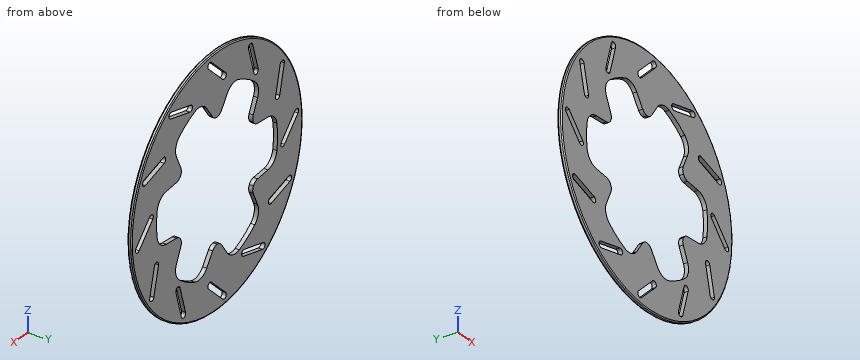
```python
from build123d import *

# Parameters (mm, degrees)
F0_R     = 120
F1_DEPTH = 4
F2_R     = 1
F3_R     = 1


# Not quite as in the source:
# - ends of sketch curves that miss each other by under 0.0002 mm in the source are joined


with BuildPart() as f1:
    # F0 (on Front) → F1 (new body)
    with BuildSketch(Plane.XZ):
        with Locations((0.769432, 5.271099)):
            Circle(F0_R)
        with BuildLine():
            ThreePointArc((-62.9582121085, -89.2513825538), (-66.5821895538, -87.0453028915), (-64.3761098915, -83.4213254462))
            Line((-64.3761098915, -83.4213254462), (-37.509664, -76.887277))
            ThreePointArc((-37.509664, -76.887277), (-33.8856864462, -79.0933561085), (-36.0917661085, -82.7173335538))
            Line((-36.0917661085, -82.7173335538), (-62.9582121085, -89.2513825538))
        make_face(mode=Mode.SUBTRACT)
        with BuildLine():
            ThreePointArc((-101.6815671027, -44.7239493504), (-103.7169843504, -41.0014398973), (-99.9944748973, -38.9660226496))
            Line((-99.9944748973, -38.9660226496), (-73.460425, -46.740593))
            ThreePointArc((-73.460425, -46.740593), (-71.4250076496, -50.4631031027), (-75.1475171027, -52.4985203504))
            Line((-75.1475171027, -52.4985203504), (-101.6815671027, -44.7239493504))
        make_face(mode=Mode.SUBTRACT)
        with BuildLine():
            ThreePointArc((-112.9532601885, 13.1996168201), (-112.8547281799, 17.4411131885), (-108.6132318115, 17.3425811799))
            Line((-108.6132318115, 17.3425811799), (-89.521356, -2.657419))
            ThreePointArc((-89.521356, -2.657419), (-89.6198878201, -6.8989151885), (-93.8613841885, -6.8003831799))
            Line((-93.8613841885, -6.8003831799), (-112.9532601885, 13.1996168201))
        make_face(mode=Mode.SUBTRACT)
        with BuildLine():
            ThreePointArc((-7.1590858201, -108.4515931885), (-11.4005821885, -108.3530611799), (-11.3020501799, -104.1115648115))
            Line((-11.3020501799, -104.1115648115), (8.69795, -85.019689))
            ThreePointArc((8.69795, -85.019689), (12.9394461885, -85.1182218201), (12.8409141799, -89.3597181885))
            Line((12.8409141799, -89.3597181885), (-7.1590858201, -108.4515931885))
        make_face(mode=Mode.SUBTRACT)
        with BuildLine():
            ThreePointArc((50.7644803504, -97.1799001027), (47.0419708973, -99.2153173504), (45.0065536496, -95.4928078973))
            Line((45.0065536496, -95.4928078973), (52.781124, -68.958759))
            ThreePointArc((52.781124, -68.958759), (56.5036341027, -66.9233416496), (58.5390513504, -70.6458511027))
            Line((58.5390513504, -70.6458511027), (50.7644803504, -97.1799001027))
        make_face(mode=Mode.SUBTRACT)
        with BuildLine():
            ThreePointArc((95.2919145538, -58.4565451085), (93.0858348915, -62.0805225538), (89.4618574462, -59.8744428915))
            Line((89.4618574462, -59.8744428915), (82.927808, -33.007997))
            ThreePointArc((82.927808, -33.007997), (85.1338871085, -29.3840194462), (88.7578645538, -31.5900991085))
            Line((88.7578645538, -31.5900991085), (95.2919145538, -58.4565451085))
        make_face(mode=Mode.SUBTRACT)
        with BuildLine():
            ThreePointArc((114.4921251885, -2.6574188201), (114.3935931799, -6.8989151885), (110.1520968115, -6.8003831799))
            Line((110.1520968115, -6.8003831799), (91.060221, 13.199617))
            ThreePointArc((91.060221, 13.199617), (91.1587528201, 17.4411131885), (95.4002491885, 17.3425811799))
            Line((95.4002491885, 17.3425811799), (114.4921251885, -2.6574188201))
        make_face(mode=Mode.SUBTRACT)
        with BuildLine():
            ThreePointArc((-93.7530495538, 68.9987431085), (-91.5469698915, 72.6227205538), (-87.9229924462, 70.4166408915))
            Line((-87.9229924462, 70.4166408915), (-81.388943, 43.550195))
            ThreePointArc((-81.388943, 43.550195), (-83.5950221085, 39.9262174462), (-87.2189995538, 42.1322971085))
            Line((-87.2189995538, 42.1322971085), (-93.7530495538, 68.9987431085))
        make_face(mode=Mode.SUBTRACT)
        with BuildLine():
            ThreePointArc((-49.2256163504, 107.7220981027), (-45.5031068973, 109.7575153504), (-43.4676896496, 106.0350058973))
            Line((-43.4676896496, 106.0350058973), (-51.24226, 79.500956))
            ThreePointArc((-51.24226, 79.500956), (-54.9647691027, 77.4655396496), (-57.0001863504, 81.1880491027))
            Line((-57.0001863504, 81.1880491027), (-49.2256163504, 107.7220981027))
        make_face(mode=Mode.SUBTRACT)
        with BuildLine():
            ThreePointArc((15.296097835, 79.396963116), (22.7229925826, 84.7551105395), (31.8731110928, 84.3758472359))
            ThreePointArc((31.8731110928, 84.3758472359), (43.2694321028, 78.8832582623), (53.724314001, 71.7600490012))
            ThreePointArc((53.724314001, 71.7600490012), (58.6278254217, 64.0254452963), (57.7009806311, 54.9144921712))
            Line((57.7009806311, 54.9144921712), (51.557275, 41.678832))
            ThreePointArc((51.557275, 41.678832), (50.8675495212, 38.1873960638), (51.8649313537, 34.7710992042))
            ThreePointArc((51.8649313537, 34.7710992042), (54.3248400002, 32.1991927067), (57.6933760416, 31.0507944662))
            Line((57.6933760416, 31.0507944662), (72.227646, 29.753569))
            ThreePointArc((72.227646, 29.753569), (80.5813855597, 26.0007639127), (84.8279934344, 17.8868970652))
            ThreePointArc((84.8279934344, 17.8868970652), (85.769432, 5.271099), (84.8279927873, -7.3446989681))
            ThreePointArc((84.8279927873, -7.3446989681), (80.5813855597, -15.4585659127), (72.2276460446, -19.2113714997))
            Line((72.2276460446, -19.2113714997), (57.693376, -20.508597))
            ThreePointArc((57.693376, -20.508597), (54.3248400002, -21.6569947067), (51.8649313537, -24.2289012042))
            ThreePointArc((51.8649313537, -24.2289012042), (50.8675495212, -27.6451980638), (51.5572758618, -31.1366350642))
            Line((51.5572758618, -31.1366350642), (57.700981, -44.372294))
            ThreePointArc((57.700981, -44.372294), (58.6278254217, -53.4832472963), (53.7243149172, -61.217850896))
            ThreePointArc((53.7243149172, -61.217850896), (43.2694321028, -68.3410602623), (31.8731109925, -73.833648981))
            ThreePointArc((31.8731109925, -73.833648981), (22.7229925826, -74.2129125395), (15.296097835, -68.854765116))
            Line((15.296097835, -68.854765116), (6.905533, -56.91633))
            ThreePointArc((6.905533, -56.91633), (4.2267227516, -54.5732912865), (0.769432, -53.728901))
            ThreePointArc((0.769432, -53.728901), (-2.6878587516, -54.5732912865), (-5.3666687757, -56.9163301576))
            Line((-5.3666687757, -56.9163301576), (-13.757233, -68.854765))
            ThreePointArc((-13.757233, -68.854765), (-21.1841275826, -74.2129125395), (-30.3342460928, -73.8336492359))
            ThreePointArc((-30.3342460928, -73.8336492359), (-41.7305681028, -68.3410602623), (-52.185450001, -61.2178510012))
            ThreePointArc((-52.185450001, -61.2178510012), (-57.0889604217, -53.4832472963), (-56.1621156311, -44.3722941712))
            Line((-56.1621156311, -44.3722941712), (-50.018411, -31.136635))
            ThreePointArc((-50.018411, -31.136635), (-49.3286845212, -27.6451980638), (-50.3260663537, -24.2289012042))
            ThreePointArc((-50.3260663537, -24.2289012042), (-52.7859750002, -21.6569947067), (-56.1545110416, -20.5085964662))
            Line((-56.1545110416, -20.5085964662), (-70.688781, -19.211372))
            ThreePointArc((-70.688781, -19.211372), (-79.0425205597, -15.4585659127), (-83.2891284344, -7.3446990652))
            ThreePointArc((-83.2891284344, -7.3446990652), (-84.230568, 5.271099), (-83.2891287873, 17.8868969681))
            ThreePointArc((-83.2891287873, 17.8868969681), (-79.0425205597, 26.0007639127), (-70.6887810446, 29.7535694997))
            Line((-70.6887810446, 29.7535694997), (-56.154511, 31.050794))
            ThreePointArc((-56.154511, 31.050794), (-52.7859750002, 32.1991927067), (-50.3260663537, 34.7710992042))
            ThreePointArc((-50.3260663537, 34.7710992042), (-49.3286845212, 38.1873960638), (-50.0184108618, 41.6788330642))
            Line((-50.0184108618, 41.6788330642), (-56.162116, 54.914492))
            ThreePointArc((-56.162116, 54.914492), (-57.0889604217, 64.0254452963), (-52.1854499172, 71.760048896))
            ThreePointArc((-52.1854499172, 71.760048896), (-41.7305681028, 78.8832582623), (-30.3342469925, 84.375846981))
            ThreePointArc((-30.3342469925, 84.375846981), (-21.1841275826, 84.7551105395), (-13.757232835, 79.396963116))
            Line((-13.757232835, 79.396963116), (-5.366668, 67.458528))
            ThreePointArc((-5.366668, 67.458528), (-2.6878587516, 65.1154892865), (0.769432, 64.271099))
            ThreePointArc((0.769432, 64.271099), (4.2267227516, 65.1154892865), (6.9055327757, 67.4585281576))
            Line((6.9055327757, 67.4585281576), (15.296097835, 79.396963116))
        make_face(mode=Mode.SUBTRACT)
        with BuildLine():
            ThreePointArc((103.2204321027, 55.2661473504), (105.2558493504, 51.5436378973), (101.5333398973, 49.5082206496))
            Line((101.5333398973, 49.5082206496), (74.99929, 57.282791))
            ThreePointArc((74.99929, 57.282791), (72.9638726496, 61.0053001027), (76.6863821027, 63.0407173504))
            Line((76.6863821027, 63.0407173504), (103.2204321027, 55.2661473504))
        make_face(mode=Mode.SUBTRACT)
        with BuildLine():
            ThreePointArc((64.4970771085, 99.7935805538), (68.1210545538, 97.5875008915), (65.9149748915, 93.9635234462))
            Line((65.9149748915, 93.9635234462), (39.048529, 87.429474))
            ThreePointArc((39.048529, 87.429474), (35.4245514462, 89.6355541085), (37.6306311085, 93.2595315538))
            Line((37.6306311085, 93.2595315538), (64.4970771085, 99.7935805538))
        make_face(mode=Mode.SUBTRACT)
        with BuildLine():
            ThreePointArc((8.6979498201, 118.9937911885), (12.9394461885, 118.8952591799), (12.8409141799, 114.6537628115))
            Line((12.8409141799, 114.6537628115), (-7.159085, 95.561887))
            ThreePointArc((-7.159085, 95.561887), (-11.4005821885, 95.6604188201), (-11.3020501799, 99.9019151885))
            Line((-11.3020501799, 99.9019151885), (8.6979498201, 118.9937911885))
        make_face(mode=Mode.SUBTRACT)
    extrude(amount=F1_DEPTH)

    # F2
    f2_edges = [f1.edges().sort_by_distance(p)[0] for p in [
        (-119.230568, -4, 5.271099),
    ]]
    fillet(f2_edges, radius=F2_R)

    # F3
    f3_edges = [f1.edges().sort_by_distance(p)[0] for p in [
        (-119.230568, 0, 5.271099),
    ]]
    fillet(f3_edges, radius=F3_R)


solid = f1.part
```
Work out the finished part from the listing and answer in its coordinate system (mm). Round coordinates to 2 decimals unless told otherwise and drop trailing zeros. Return JSON: item names as keys, results as strings. Group by question number.
Q1. Find the intervals of material crossed by L1, parallel to Z at x = 39.5, y = -1.8; L2, parallel to X at y = -2.15, z = -33.5; L3, parallel to Z at x = 65.5, y = -2.6, in increasing order.
Q2. The part is cut by section A-A on z = -80. Count the separate pieces of the cut face and the enclosed holes in it, then the cut area to 3 significant figures.
Q3. Each of these flat-tipped pins is pushed along its axis until it touches: pin 1 Ø2 at (y, z) = (-1, 88) entering from -X; pin 2 Ø2 at (x, y) = (89, -3) entering from +Z. Where does it stop, or does it pass through?
Solved:
{
 "1": {"L1": "-108.31 to -70.39, 80.93 to 87.54, 93.71 to 118.85", "L2": "-112.79 to -51.12, 52.65 to 83.05, 89.22 to 114.33", "L3": "-95.77 to -19.81, 30.35 to 93.86, 99.86 to 106.32"},
 "2": {"separate pieces": "3", "enclosed holes": "0", "area": "583 mm²"},
 "3": {"pin 1": "x = -87.1", "pin 2": "z = 87.68"}
}
